Geometry check sheet. Reference: the model listing, model coordinates, mm. Give positions to 0.01 mm unless a question says otherwise; leave off trailing zeros. Loops run counter-clockwise (first coordinate to the right, second up) from the corner with the lowest first, then second, coordinate; pieces in that order, holes last. Notation, with made-up numbers: (-38.5, 16.5) - (-2.5, 16.5) arc R15 cw to (-2.5, 37.5) - close; hole circle Ø8 at (-2, 29). An arc over 180 degrees is marked (long way). Use a Markdown table: item, result. Add a question column.
1. Depth check by flat-ended pin: P1, Ø1.5, axis at x = -1.5, y = 14, coming from the +Z side; P2, Ø1.5, axis at x = -0.5, z = 4, coming from the -Y side; P3, Ø1, axis at y = 5.5, z = -1.5, coming from the +X side. Enter the tip coordinate at first touch or a pass-through.
2. Cross-section at C-C on y = 14.75. Enter the section's corners in (x, z).
3. Cross-section at D-D on y = 18.25. Enter the section's corners in (x, z).
4. Material ranges on L1, parallel to Z at x = 0, y = 9; L2, parallel to X at y = 17.25, z = -4, recorded low to high.
5. Cross-section at A-A on x = 0. Enter the section's corners in (y, z).
6. Draft check along Y on faces 1 (the cylindrical face through (5.95, 9.86, -0.78)), 2 (the flat face through (2, 0, 6)), 3 (the cylindrical face through (-3.2, 17.6, -5.5)), 4 (the cylindrical face through (-0.521, 23.966, 5.437)). Enter one of: pulls with the +Y half, pulls with the -Y half, needs draft (parallel to the pull), parting line crosses it, or undercut.
7. Cross-section at B-B on z = 0. Enter the section's corners in (x, y), and give its area (3 significant figures).
from build123d import *

# Parameters (mm, degrees)
SKETCH_1_R               = 7
SKETCH_1_R_2             = 6
EXTRUDE_1_DEPTH          = 20
CUT_EXTRUDE_1_DEPTH      = 29.757607689
CUT_EXTRUDE_1_DEPTH_BACK = 29.757607689
SKETCH_3_R               = 4


with BuildPart() as part:
    # 草图1 → 凸台-拉伸1 (new body)
    with BuildSketch(Plane(origin=(0, 0, 0), x_dir=(1, 0, 0), z_dir=(0, 1, 0))):
        with Locations(Location((0, 0, 0), (0, 0, 270))):
            Circle(SKETCH_1_R)
        with Locations(Location((0, 0, 0), (0, 0, 270))):
            Circle(SKETCH_1_R_2, mode=Mode.SUBTRACT)
    extrude(amount=EXTRUDE_1_DEPTH)

    # 草图2 → 旋转1 (revolve)
    with BuildSketch(Plane.XY):
        with BuildLine():
            Line((-7, 20), (-6, 20))
            ThreePointArc((-6, 20), (-4.242640687, 24.242640687), (0, 26))
            Line((0, 26), (0, 27))
            ThreePointArc((0, 27), (-4.949747468, 24.949747468), (-7, 20))
        make_face()
    revolve(axis=Axis((0, 20, 0), (0, 1, 0)))

    # 草图3 → 切除-拉伸1 (cut, two sides: drawn at the far end of the back side and taken through both)
    with BuildSketch(Plane.XY.offset(-CUT_EXTRUDE_1_DEPTH_BACK)):
        with Locations((0, 20)):
            Circle(SKETCH_3_R)
    extrude(amount=CUT_EXTRUDE_1_DEPTH + CUT_EXTRUDE_1_DEPTH_BACK, mode=Mode.SUBTRACT)


solid = part.part
Values found:
| question | item | result |
|---|---|---|
| 1 | P1 | stops at z = 6.96 |
| 1 | P2 | stops at y = 23.85 |
| 1 | P3 | stops at x = 6.93 |
| 2 | outline | circle Ø14 at (0, 0); hole circle Ø12 at (0, 0) |
| 3 | outline | (-3.6, -6.01) - (-3.6, -4.8) arc R6 cw to (-3.6, 4.8) - (-3.6, 6.01) arc R7 ccw to start; (3.6, -6.01) arc R7 ccw to (3.6, 6.01) - (3.6, 4.8) arc R6 cw to (3.6, -4.8) - close |
| 4 | L1 | z = -7 to -6, 6 to 7 |
| 4 | L2 | x = -5.74 to -4.47, 4.47 to 5.74 |
| 5 | outline | (0, -7) - (16, -7) - (16, -6) - (0, -6) - close; (0, 6) - (16, 6) - (16, 7) - (0, 7) - close; (24, -5.74) arc R7 ccw to (24, 5.74) - (24, 4.47) arc R6 cw to (24, -4.47) - close |
| 6 | face 1 | needs draft |
| 6 | face 2 | pulls with the -Y half |
| 6 | face 3 | undercut |
| 6 | face 4 | undercut |
| 7 | outline | (-7, 0) - (-6, 0) - (-6, 20) arc R6 cw to (6, 20) - (6, 0) - (7, 0) - (7, 20) arc R7 ccw to (-7, 20) - close |
| 7 | area | 60.4 mm2 |
